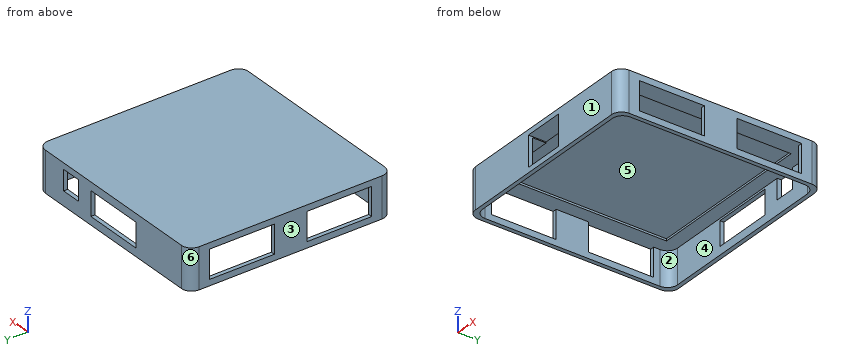
```python
from build123d import *

# Parameters (mm, degrees)
SKETCH_2_W          = 100
SKETCH_2_H          = 100
EXTRUDE_1_DEPTH     = 20
SKETCH_3_W          = 10
SKETCH_3_H          = 10
CUT_EXTRUDE_1_DEPTH = 12
SKETCH_4_W          = 96
SKETCH_4_H          = 96
CUT_EXTRUDE_2_DEPTH = 17
SKETCH_5_W          = 82.5
SKETCH_5_H          = 82.5
CUT_EXTRUDE_3_DEPTH = 1
FILLET_1_R          = 5
FILLET_2_R          = 5
SKETCH_8_W          = 14
SKETCH_8_H          = 32
CUT_EXTRUDE_4_DEPTH = 114.578166916
SKETCH_9_W          = 20
SKETCH_9_H          = 15
CUT_EXTRUDE_5_DEPTH = 10
SKETCH_10_W         = 30
SKETCH_10_H         = 12
CUT_EXTRUDE_6_DEPTH = 10


with BuildPart() as part:
    # 草图2 → 凸台-拉伸1 (new body)
    with BuildSketch(Plane.XY):
        Rectangle(SKETCH_2_W, SKETCH_2_H)
    extrude(amount=EXTRUDE_1_DEPTH)

    # 草图3 → 切除-拉伸1 (cut)
    with BuildSketch(Plane(origin=(0, 50, 0), x_dir=(1, 0, 0), z_dir=(0, 1, 0))):
        with Locations((28, -12)):
            Rectangle(SKETCH_3_W, SKETCH_3_H)
    extrude(amount=-CUT_EXTRUDE_1_DEPTH, mode=Mode.SUBTRACT)

    # 草图4 → 切除-拉伸2 (cut)
    with BuildSketch(Plane(origin=(0, 0, 0), x_dir=(-1, 0, 0), z_dir=(0, 0, -1))):
        Rectangle(SKETCH_4_W, SKETCH_4_H)
    extrude(amount=-CUT_EXTRUDE_2_DEPTH, mode=Mode.SUBTRACT)

    # 草图5 → 切除-拉伸3 (cut)
    with BuildSketch(Plane(origin=(0, 0, 17), x_dir=(-1, 0, 0), z_dir=(0, 0, -1))):
        Rectangle(SKETCH_5_W, SKETCH_5_H)
    extrude(amount=-CUT_EXTRUDE_3_DEPTH, mode=Mode.SUBTRACT)

    # 圆角1
    fillet_1_edges = [part.edges().sort_by_distance(p)[0] for p in [
        (48, 48, 8.5),
        (-48, 48, 8.5),
        (-48, -48, 8.5),
        (48, -48, 8.5),
    ]]
    fillet(fillet_1_edges, radius=FILLET_1_R)

    # 圆角2
    fillet_2_edges = [part.edges().sort_by_distance(p)[0] for p in [
        (50, -50, 10),
        (-50, -50, 10),
        (-50, 50, 10),
        (50, 50, 10),
    ]]
    fillet(fillet_2_edges, radius=FILLET_2_R)

    # 草图8 → 切除-拉伸4 (cut, through all)
    with BuildSketch(Plane.ZY.offset(50)):
        with Locations((10, -24)):
            Rectangle(SKETCH_8_W, SKETCH_8_H)
        with Locations((10, 24)):
            Rectangle(SKETCH_8_W, SKETCH_8_H)
    extrude(amount=-CUT_EXTRUDE_4_DEPTH, mode=Mode.SUBTRACT)

    # 草图9 → 切除-拉伸5 (cut)
    with BuildSketch(Plane.XZ.offset(50)):
        with Locations((0, 10)):
            Rectangle(SKETCH_9_W, SKETCH_9_H)
    extrude(amount=-CUT_EXTRUDE_5_DEPTH, mode=Mode.SUBTRACT)

    # 草图10 → 切除-拉伸6 (cut)
    with BuildSketch(Plane(origin=(0, 50, 0), x_dir=(1, 0, 0), z_dir=(0, 1, 0))):
        with Locations((0, -10)):
            Rectangle(SKETCH_10_W, SKETCH_10_H)
    extrude(amount=-CUT_EXTRUDE_6_DEPTH, mode=Mode.SUBTRACT)


solid = part.part
```
Build history of the part. All positions in model axes, mm. Face numbers are marked on the shaded views. A direction names the side the tool comes from. Give positions to 0.01 mm unless a question says otherwise; leave off trailing zeros. Loops run counter-clockwise (first coordinate to the right, second up) from the corner with the lowest first, then second, coordinate; pieces in that order, holes last. Notation, with made-up numbers: (20.25, 75.5) - (71.25, 75.5) arc R6 cw to (71.25, 83.5) - close; hole circle Ø8 at (64.25, 53). An arc over 180 degrees is marked (long way). Use a Markdown table: item, result.
(1) Pull direction Y, two halves, no side cores. Call the marked faces 3, 4, 5 and 6: +Y half, -Y half, draft (parallel to the pull), parting line (faces both ways), or undercut.
Taken from the geometry:
| item | result |
|---|---|
| face 3 | draft |
| face 4 | undercut |
| face 5 | undercut |
| face 6 | +Y half |
(2) Band-saw the part on A-A (y = -38.5). Give the cut face in (x, z).
Taken from the geometry:
| item | result |
|---|---|
| outline | (-50, 0) - (-48, 0) - (-48, 3) - (-50, 3) - close; (-50, 17) - (-41.25, 17) - (-41.25, 18) - (41.25, 18) - (41.25, 17) - (50, 17) - (50, 20) - (-50, 20) - close; (48, 0) - (50, 0) - (50, 3) - (48, 3) - close |
(3) Which spindle directions (+Z, -Z, +X, -X, +Y, -Y) get a long thin tool onto all of the face, cutting with end or side? Do the marked faces 1 and 2. Say none if no direction does.
Taken from the geometry:
| item | result |
|---|---|
| face 1 | +Z, -Z, +X, -X, -Y |
| face 2 | -Z |
(4) Wall check: line 1 along Y through (x, z) = (-43.5, 6.5); line 2 along X through (y, z) = (-4.5, 15); line 3 along Z through (x, y) = (4.5, 6.5). Give the ranges that are in metal, low to high.
Taken from the geometry:
| item | result |
|---|---|
| line 1 | -50 to -47.97, 47.97 to 50 |
| line 2 | -50 to -48, 48 to 50 |
| line 3 | 18 to 20 |
(5) Band-saw the part on D-D (z = 8.5). Give the number of separate pieces and of enclosed holes in the cut face, and give its area (3 significant figures).
Taken from the geometry:
| item | result |
|---|---|
| separate pieces | 7 |
| enclosed holes | 0 |
| area | 408 mm2 |
(6) Drop flat-ended pins along their axis: pin 1 Ø5 at (x, y) = (-26, 3) entering from -Z; pin 2 Ø5 at (x, z) = (6, 6) entering from +Y; pin 3 Ø1.6 at (x, z) = (48.5, 12) entering from +Y; pin 4 Ø0.6 at (x, z) = (-49, 8.5) entering from +Y. Give the stop position or say it passes through.
Taken from the geometry:
| item | result |
|---|---|
| pin 1 | z = 18 |
| pin 2 | y = 50 |
| pin 3 | y = 49.21 |
| pin 4 | y = 48.36 |
(7) Band-saw the part on B-B (x = -29.5). Give the cut face in (y, z), and give its area (4 significant figures).
Taken from the geometry:
| item | result |
|---|---|
| outline | (-50, 0) - (-48, 0) - (-48, 17) - (-41.25, 17) - (-41.25, 18) - (41.25, 18) - (41.25, 17) - (48, 17) - (48, 0) - (50, 0) - (50, 20) - (-50, 20) - close |
| area | 285.5 mm2 |
